from build123d import *

# Parameters (mm, degrees)
EXTRUDE001_DEPTH = 50.25
SKETCH_W         = 100.5
SKETCH_H         = 100.5
EXTRUDE_DEPTH    = 15
SKETCH002_W      = 15
SKETCH002_H      = 30
EXTRUDE002_DEPTH = 55.25
FILLET_R         = 1


with BuildPart() as extrude001:
    # Sketch001 (on Sketch) → Extrude001 (new body, symmetric)
    with BuildSketch(Plane.YZ):
        Polygon((-55.25, 0), (-55.25, 30), (-45.25, 30), (-45.25, 15.9), (-50.25, 15.9), (-50.25, 15), (-45.25, 15), (-45.25, 0), align=None)
        Polygon((55.25, 0), (55.25, 30), (45.25, 30), (45.25, 15.9), (50.25, 15.9), (50.25, 15), (45.25, 15), (45.25, 0), align=None)
    extrude(amount=EXTRUDE001_DEPTH, both=True)


with BuildPart() as fusion:
    # Sketch → Extrude (new body)
    with BuildSketch(Plane.XY):
        Rectangle(SKETCH_W, SKETCH_H)
    extrude(amount=EXTRUDE_DEPTH)

    # Fusion: union Extrude001
    add(extrude001.part)


with BuildPart() as fillet_body:
    # Sketch002 → Extrude002 (new body, symmetric)
    with BuildSketch(Plane.XZ):
        with Locations((-42.75, -15)):
            Rectangle(SKETCH002_W, SKETCH002_H)
    extrude(amount=EXTRUDE002_DEPTH, both=True)

    # Fusion001: union Fusion
    add(fusion.part)

    # Fillet
    fillet_edges = [fillet_body.edges().sort_by_distance(p)[0] for p in [
        (-35.25, 0, 0),
        (-35.25, 0, -30),
        (-35.25, 55.25, -15),
        (-35.25, -55.25, -15),
        (-50.25, 0, -30),
        (-42.75, 55.25, -30),
        (-42.75, -55.25, -30),
        (50.25, 0, 0),
        (7.5, -55.25, 0),
        (7.5, 55.25, 0),
        (-50.25, 55.25, 0),
        (0, 55.25, 30),
        (50.25, 55.25, 15),
        (0, 45.25, 30),
        (50.25, 45.25, 22.95),
        (-50.25, 45.25, 22.95),
        (50.25, 50.25, 30),
        (-50.25, 50.25, 30),
        (50.25, -55.25, 15),
        (0, -55.25, 30),
        (-50.25, -55.25, 0),
        (0, -45.25, 30),
        (50.25, -50.25, 30),
        (-50.25, -50.25, 30),
        (50.25, -45.25, 22.95),
        (-50.25, -45.25, 22.95),
    ]]
    fillet(fillet_edges, radius=FILLET_R)


solid = fillet_body.part
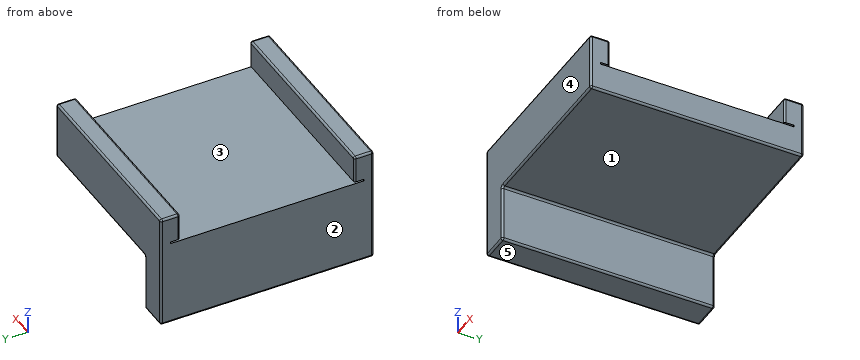
Here's how the part is built. I have some questions about the finished solid (model axes, mm). Face numbers are marked on the shaded views. A direction names the side the tool comes from. Give positions to 0.01 mm unless a question says otherwise; leave off trailing zeros. Order: outer loops, then holes, each group sorted by start corner. A loop starts at its lowest first (then second) coordinate and runs counter-clockwise, first axis right, second up. Notation, with made-up numbers: (83.25, 66) -> (122.25, 66) arc R30 ccw to (122.25, 88) -> close; hole circle Ø10 at (-35, 41.5). An arc over 180 degrees is marked (long way). Use a Markdown table: item, result. Add a question column.
Item 1: If we mould it in two halves opening along Y, with no side actions, what happens to the marked faces 3, 4 and 5? For each: pulls with the +Y half, pulls with the -Y half, needs draft (parallel to the pull), parting line crosses it, or undercut.
Item 2: I need wall thicknesses on line 1 (Y direction, x = 0.5, z = 24); line 2 (Z direction, x = -28.5, y = 48); line 3 (Z direction, x = 6.5, y = 5.5). Which ranges of each line are inside material? Lowest first, please.
Item 3: Imagine slicing it at D-D on x = 25.5. Please give me the cut outline in (y, z).
Item 4: Imagine slicing it at A-A on z = -9. Please give me the cut outline in (x, y).
Item 5: Imagine slicing it at C-C on z = 20.5. Please give me the cut outline in (x, y), plus the area to 3 significant figures.
Item 6: Will these pins go through, and if not, where does the flat tip stop? pin 1 (5.5 mm diameter, centred on x = -23, y = -47, fed in from -Z); pin 2 (10 mm diameter, centred on x = 2, y = 20, fed in from +Z); pin 3 (10 mm diameter, centred on x = 4.5, z = -4.5, fed in from +Y).
Item 7: Imagine slicing it at B-B on y = -17.5. Please give me the cut outline in (x, z), plus the area to 3 significant figures.
Item 8: For the marked faces 1 and 2, which set-ups out of +Z, -Z, +X, -X, +Y, -Y let a thin tool reach every point of the face, with its end or its side?
Data:
| question | item | result |
|---|---|---|
| 1 | face 3 | undercut |
| 1 | face 4 | pulls with the -Y half |
| 1 | face 5 | needs draft |
| 2 | line 1 | y = -55.25 to -45.25, 45.25 to 55.25 |
| 2 | line 2 | z = 0 to 15, 15.9 to 30 |
| 2 | line 3 | z = 0 to 15 |
| 3 | outline | (-55.25, 1) arc R1 ccw to (-54.25, 0) -> (54.25, 0) arc R1 ccw to (55.25, 1) -> (55.25, 29) arc R1 ccw to (54.25, 30) -> (46.25, 30) arc R1 ccw to (45.25, 29) -> (45.25, 15.9) -> (50.25, 15.9) -> (50.25, 15) -> (-50.25, 15) -> (-50.25, 15.9) -> (-45.25, 15.9) -> (-45.25, 29) arc R1 ccw to (-46.25, 30) -> (-54.25, 30) arc R1 ccw to (-55.25, 29) -> close |
| 4 | outline | (-50.25, -54.25) arc R1 ccw to (-49.25, -55.25) -> (-36.25, -55.25) arc R1 ccw to (-35.25, -54.25) -> (-35.25, 54.25) arc R1 ccw to (-36.25, 55.25) -> (-49.25, 55.25) arc R1 ccw to (-50.25, 54.25) -> close |
| 5 | outline | (-50.25, -54.25) arc R1 ccw to (-49.25, -55.25) -> (49.25, -55.25) arc R1 ccw to (50.25, -54.25) -> (50.25, -46.25) arc R1 ccw to (49.25, -45.25) -> (-49.25, -45.25) arc R1 ccw to (-50.25, -46.25) -> close; (-50.25, 46.25) arc R1 ccw to (-49.25, 45.25) -> (49.25, 45.25) arc R1 ccw to (50.25, 46.25) -> (50.25, 54.25) arc R1 ccw to (49.25, 55.25) -> (-49.25, 55.25) arc R1 ccw to (-50.25, 54.25) -> close |
| 5 | area | 2,010 mm² |
| 6 | pin 1 | stops at z = 0 |
| 6 | pin 2 | stops at z = 15 |
| 6 | pin 3 | stops at y = 55.12 |
| 7 | outline | (-50.25, -29) arc R1 ccw to (-49.25, -30) -> (-36.25, -30) arc R1 ccw to (-35.25, -29) -> (-35.25, -1) arc R1 cw to (-34.25, 0) -> (49.25, 0) arc R1 ccw to (50.25, 1) -> (50.25, 15) -> (-50.25, 15) -> close |
| 7 | area | 1,960 mm² |
| 8 | face 1 | -Z, +X, +Y, -Y |
| 8 | face 2 | +Z, -Z, -X, +Y, -Y |
